The model under review builds one solid part; all positions refer to its coordinate system, in mm. A direction names the side the tool comes from. Coordinates: 2 decimals unless noted, no trailing zeros. Order: outer loops, then holes, each group sorted by start corner. A loop starts at its lowest first (then second) coordinate and runs counter-clockwise, first axis right, second up. Notation, with made-up numbers: M 82.5,83 L 121.5,83 A19 ccw 121.5,115 Z; hole C 88,64 d10. An arc over 180 degrees is marked long. One line per item, written item: value.
```python
from build123d import *

# Parameters (mm, degrees)
SKETCH1_R           = 3.5
BOSS_EXTRUDE1_DEPTH = 4
CUT_EXTRUDE1_DEPTH  = 2.25
CHAMFER1_SIZE       = 0.35
SKETCH_1_R          = 2
EXTRUDE_1_DEPTH     = 30


with BuildPart() as part:
    # Sketch1 → Boss-Extrude1 (new body)
    with BuildSketch(Plane(origin=(0, 0, 0), x_dir=(1, 0, 0), z_dir=(0, 1, 0))):
        with Locations(Location((0, 0, 0), (0, 0, 270))):
            Circle(SKETCH1_R)
    extrude(amount=BOSS_EXTRUDE1_DEPTH)

    # Sketch2 → Cut-Extrude1 (cut)
    with BuildSketch(Plane(origin=(0, 4, 0), x_dir=(1, 0, 0), z_dir=(0, 1, 0))):
        Polygon((0.866025404, 1.5), (-0.866025404, 1.5), (-1.732050808, 0), (-0.866025404, -1.5), (0.866025404, -1.5), (1.732050808, 0), align=None)
    extrude(amount=-CUT_EXTRUDE1_DEPTH, mode=Mode.SUBTRACT)

    # Cut-Extrude2 cone 1 section (through the dimple's axis) → Cut-Extrude2 (revolve, cut)
    with BuildSketch(Plane(origin=(0, 4, 0), x_dir=(0, 0, 1), z_dir=(1, 0, 0))):
        Polygon((0, 0), (1.732050808, 0), (0, 1.732050808), align=None)
    revolve(axis=Axis((0, 4, 0), (0, -1, 0)), mode=Mode.SUBTRACT)

    # Chamfer1
    chamfer1_edges = [part.edges().sort_by_distance(p)[0] for p in [
        (0, 0, -3.5),
        (0, 4, -3.5),
    ]]
    chamfer(chamfer1_edges, length=CHAMFER1_SIZE)

    # 草图1 → 凸台-拉伸1 (add)
    with BuildSketch(Plane(origin=(0, 0, 0), x_dir=(-1, 0, 0), z_dir=(0, -1, 0))):
        with Locations(Location((0, 0, 0), (0, 0, 90))):
            Circle(SKETCH_1_R)
    extrude(amount=EXTRUDE_1_DEPTH)


solid = part.part
```
(1) Insertion check: pin 1 Ø2 at (x, y) = (2, -19.5) entering from -Z; pin 2 Ø2 at (x, y) = (0, -21.5) entering from +Z; pin 3 Ø0.5 at (x, y) = (-0.5, 2.5) entering from -Z. Each pin has a flat end and moves straight along its axis. Give the tip position at first contact, or say it passes through.
Geometry results:
pin 1: stops at z = -1.73
pin 2: stops at z = 2
pin 3: stops at z = -3.49
(2) Tool access review of faces 5 (the flat face through (-2, 0, 1)), 6 (the flat face through (0, 3, 1.5)), 7 (the flat face through (0, -30, 0)): name each direction out of +Z, -Z, +X, -X, +Y, -Y from which nothing blocks a thin tool from reaching the whole face with its end or side.
Geometry results:
face 5: -Y
face 6: +Y
face 7: +Z, -Z, +X, -X, -Y
(3) We need section A-A, the plane x = 0. State the section outline as (y, z) points, plus the area to 3 significant figures.
Geometry results:
outline: M -30,-2 L 0,-2 L 0,-3.15 L 0.35,-3.5 L 3.65,-3.5 L 4,-3.15 L 4,-1.73 L 3.77,-1.5 L 1.75,-1.5 L 1.75,1.5 L 3.77,1.5 L 4,1.73 L 4,3.15 L 3.65,3.5 L 0.35,3.5 L 0,3.15 L 0,2 L -30,2 Z
area: 141 mm2
(4) We need section B-B, the plane y = -7. State the section outline as (x, z) points.
Geometry results:
outline: C 0,0 d4
(5) Mouldability with a two-part tool opening along X and no side actions: class faces 1 (the flat face through (1.305, 2.891, -0.74)), 2 (the cylindrical face through (-2, -15, 0)), 3 (the flat face through (-1.293, 2.891, -0.761)), 4 (the flat face through (-1.4, 4, 1.4)) as +X half, -X half, draft (parallel to the pull), parting line (faces both ways), or undercut.
Geometry results:
face 1: undercut
face 2: parting line
face 3: undercut
face 4: draft
(6) For L1, parallel to Y at x = 0.5, z = 2; L2, parallel to Z at x = -1, y = -12.5; L3, parallel to Y at x = 0.75, z = -1, list the stretches that pass through material, from the lowest coordinate up.
Geometry results:
L1: y = 0 to 4
L2: z = -1.73 to 1.73
L3: y = -30 to 1.75
